Can you work these out from the model? Positions are in its coordinate system, mm. Give positions to 0.01 mm unless a question says otherwise; leave off trailing zeros. Write each loop counter-clockwise with the first axis right and the second up, starting at its lowest first coordinate (ties: lowest second). Pieces come first, ordered by that corner, then holes. Notation, with made-up numbers: (50.5, 4) -> (78.5, 4) arc R20 cw to (78.5, 17) -> close; hole circle Ø11 at (5, 23). An arc over 180 degrees is marked (long way). Answer as CSV lines item,"result". Start each with the question number.
1. If we section it at B-B on x = 1.5: Write out the boundary of the cut face in (y, z), plus the area to 3 significant figures.
2. I need wall thicknesses on line 1 (X direction, y = 0.2, z = -4.5); line 2 (X direction, y = 0.25, z = -1); line 3 (Z direction, x = 0.25, y = 0.3). Which ranges of each line are inside material? Lowest first, please. Write a range as [from, to].
3. If we section it at A-A on z = 1: Write out the boundary of the cut face in (x, y).
4. If we section it at C-C on y = 0.4: Count the separate pieces of the cut face and the enclosed holes in it, plus the area to 3 significant figures.
5. If we section it at D-D on x = -4.5: Write out the boundary of the cut face in (y, z), plus the area to 3 significant figures.
```python
from build123d import *

# Parameters (mm, degrees)
ESQUISSE1_R        = 0.16
BOSS_EXTRU_1_DEPTH = 0.5


with BuildPart() as part:
    # Esquisse1 → Boss.-Extru.1 (new body)
    with BuildSketch(Plane(origin=(0, 0, 0), x_dir=(1, 0, 0), z_dir=(0, 1, 0))):
        with BuildLine():
            ThreePointArc((5.497543289, -0.164370862), (5.499385788, -0.08219461), (5.5, 0))
            ThreePointArc((5.5, 0), (5.499385788, 0.08219461), (5.497543289, 0.164370862))
            ThreePointArc((5.497543289, 0.164370862), (4.96354437, 0.602683401), (5.377131195, 1.15605368))
            ThreePointArc((5.377131195, 1.15605368), (5.340179996, 1.316236154), (5.298458151, 1.475242768))
            ThreePointArc((5.298458151, 1.475242768), (4.675081213, 1.773024435), (4.94421978, 2.409292585))
            ThreePointArc((4.94421978, 2.409292585), (4.870008141, 2.555977446), (4.791445883, 2.700378926))
            ThreePointArc((4.791445883, 2.700378926), (4.114919329, 2.840323734), (4.223968284, 3.522512163))
            ThreePointArc((4.223968284, 3.522512163), (4.116809115, 3.64717462), (4.005972198, 3.768578877))
            ThreePointArc((4.005972198, 3.768578877), (3.315613291, 3.742553741), (3.258235104, 4.431016137))
            ThreePointArc((3.258235104, 4.431016137), (3.124356107, 4.526411262), (2.987685969, 4.617762722))
            ThreePointArc((2.987685969, 4.617762722), (2.32361586, 4.427280128), (2.103145143, 5.082005559))
            ThreePointArc((2.103145143, 5.082005559), (1.950326879, 5.142589335), (1.795766291, 5.198578982))
            ThreePointArc((1.795766291, 5.198578982), (1.196578321, 4.854709087), (0.825828031, 5.437647291))
            ThreePointArc((0.825828031, 5.437647291), (0.662951741, 5.459898808), (0.499483204, 5.477272727))
            ThreePointArc((0.499483204, 5.477272727), (0, 5), (-0.499483204, 5.477272727))
            ThreePointArc((-0.499483204, 5.477272727), (-0.662951741, 5.459898808), (-0.825828031, 5.437647291))
            ThreePointArc((-0.825828031, 5.437647291), (-0.818639901, 5.389149062), (-0.816236154, 5.340179996))
            ThreePointArc((-0.816236154, 5.340179996), (-1.24469969, 4.845323921), (-1.795766291, 5.198578982))
            ThreePointArc((-1.795766291, 5.198578982), (-1.950326879, 5.142589335), (-2.103145143, 5.082005559))
            ThreePointArc((-2.103145143, 5.082005559), (-2.067911799, 4.978598768), (-2.055977446, 4.870008141))
            ThreePointArc((-2.055977446, 4.870008141), (-2.425314256, 4.387382892), (-2.987685969, 4.617762722))
            ThreePointArc((-2.987685969, 4.617762722), (-3.124356107, 4.526411262), (-3.258235104, 4.431016137))
            ThreePointArc((-3.258235104, 4.431016137), (-3.175756675, 4.283437807), (-3.14717462, 4.116809115))
            ThreePointArc((-3.14717462, 4.116809115), (-3.459290066, 3.653452455), (-4.005972198, 3.768578877))
            ThreePointArc((-4.005972198, 3.768578877), (-4.116809115, 3.64717462), (-4.223968284, 3.522512163))
            ThreePointArc((-4.223968284, 3.522512163), (-4.078515354, 3.346593042), (-4.026411262, 3.124356107))
            ThreePointArc((-4.026411262, 3.124356107), (-4.284045125, 2.687024819), (-4.791445883, 2.700378926))
            ThreePointArc((-4.791445883, 2.700378926), (-4.870008141, 2.555977446), (-4.94421978, 2.409292585))
            ThreePointArc((-4.94421978, 2.409292585), (-4.724746794, 2.224931342), (-4.642589335, 1.950326879))
            ThreePointArc((-4.642589335, 1.950326879), (-4.849275857, 1.545398238), (-5.298458151, 1.475242768))
            ThreePointArc((-5.298458151, 1.475242768), (-5.340179996, 1.316236154), (-5.377131195, 1.15605368))
            ThreePointArc((-5.377131195, 1.15605368), (-5.07820272, 0.985919382), (-4.959898808, 0.662951741))
            ThreePointArc((-4.959898808, 0.662951741), (-5.119915162, 0.296330519), (-5.497543289, 0.164370862))
            ThreePointArc((-5.497543289, 0.164370862), (-5.5, 0), (-5.497543289, -0.164370862))
            ThreePointArc((-5.497543289, -0.164370862), (-5.119915162, -0.296330519), (-4.959898808, -0.662951741))
            ThreePointArc((-4.959898808, -0.662951741), (-5.07820272, -0.985919382), (-5.377131195, -1.15605368))
            ThreePointArc((-5.377131195, -1.15605368), (-5.340179996, -1.316236154), (-5.298458151, -1.475242768))
            ThreePointArc((-5.298458151, -1.475242768), (-4.849275857, -1.545398238), (-4.642589335, -1.950326879))
            ThreePointArc((-4.642589335, -1.950326879), (-4.724746794, -2.224931342), (-4.94421978, -2.409292585))
            ThreePointArc((-4.94421978, -2.409292585), (-4.870008141, -2.555977446), (-4.791445883, -2.700378926))
            ThreePointArc((-4.791445883, -2.700378926), (-4.284045125, -2.687024819), (-4.026411262, -3.124356107))
            ThreePointArc((-4.026411262, -3.124356107), (-4.078515354, -3.346593042), (-4.223968284, -3.522512163))
            ThreePointArc((-4.223968284, -3.522512163), (-4.116809115, -3.64717462), (-4.005972198, -3.768578877))
            ThreePointArc((-4.005972198, -3.768578877), (-3.459290066, -3.653452455), (-3.14717462, -4.116809115))
            ThreePointArc((-3.14717462, -4.116809115), (-3.175756675, -4.283437807), (-3.258235104, -4.431016137))
            ThreePointArc((-3.258235104, -4.431016137), (-3.124356107, -4.526411262), (-2.987685969, -4.617762722))
            ThreePointArc((-2.987685969, -4.617762722), (-2.425314256, -4.387382892), (-2.055977446, -4.870008141))
            ThreePointArc((-2.055977446, -4.870008141), (-2.067911799, -4.978598768), (-2.103145143, -5.082005559))
            ThreePointArc((-2.103145143, -5.082005559), (-1.950326879, -5.142589335), (-1.795766291, -5.198578982))
            ThreePointArc((-1.795766291, -5.198578982), (-1.24469969, -4.845323921), (-0.816236154, -5.340179996))
            ThreePointArc((-0.816236154, -5.340179996), (-0.818639901, -5.389149062), (-0.825828031, -5.437647291))
            ThreePointArc((-0.825828031, -5.437647291), (-0.662951741, -5.459898808), (-0.499483204, -5.477272727))
            ThreePointArc((-0.499483204, -5.477272727), (0, -5), (0.499483204, -5.477272727))
            ThreePointArc((0.499483204, -5.477272727), (0.662951741, -5.459898808), (0.825828031, -5.437647291))
            ThreePointArc((0.825828031, -5.437647291), (1.196578321, -4.854709087), (1.795766291, -5.198578982))
            ThreePointArc((1.795766291, -5.198578982), (1.950326879, -5.142589335), (2.103145143, -5.082005559))
            ThreePointArc((2.103145143, -5.082005559), (2.32361586, -4.427280128), (2.987685969, -4.617762722))
            ThreePointArc((2.987685969, -4.617762722), (3.124356107, -4.526411262), (3.258235104, -4.431016137))
            ThreePointArc((3.258235104, -4.431016137), (3.315613291, -3.742553741), (4.005972198, -3.768578877))
            ThreePointArc((4.005972198, -3.768578877), (4.116809115, -3.64717462), (4.223968284, -3.522512163))
            ThreePointArc((4.223968284, -3.522512163), (4.114919329, -2.840323734), (4.791445883, -2.700378926))
            ThreePointArc((4.791445883, -2.700378926), (4.870008141, -2.555977446), (4.94421978, -2.409292585))
            ThreePointArc((4.94421978, -2.409292585), (4.675081213, -1.773024435), (5.298458151, -1.475242768))
            ThreePointArc((5.298458151, -1.475242768), (5.340179996, -1.316236154), (5.377131195, -1.15605368))
            ThreePointArc((5.377131195, -1.15605368), (4.96354437, -0.602683401), (5.497543289, -0.164370862))
        make_face()
        with Locations((0, -4)):
            Circle(ESQUISSE1_R, mode=Mode.SUBTRACT)
        with Locations((-4, 0)):
            Circle(ESQUISSE1_R, mode=Mode.SUBTRACT)
        with BuildLine():
            ThreePointArc((3.8, 0), (-2.687005769, -2.687005769), (0, 3.8))
            ThreePointArc((0, 3.8), (2.687005769, 2.687005769), (3.8, 0))
        make_face(mode=Mode.SUBTRACT)
        with BuildLine():
            ThreePointArc((0.16, 4), (0.113137085, 3.886862915), (0, 3.84))
            ThreePointArc((0, 3.84), (-0.113137085, 4.113137085), (0.16, 4))
        make_face(mode=Mode.SUBTRACT)
        with Locations((4, 0)):
            Circle(ESQUISSE1_R, mode=Mode.SUBTRACT)
    extrude(amount=BOSS_EXTRU_1_DEPTH)


solid = part.part
```
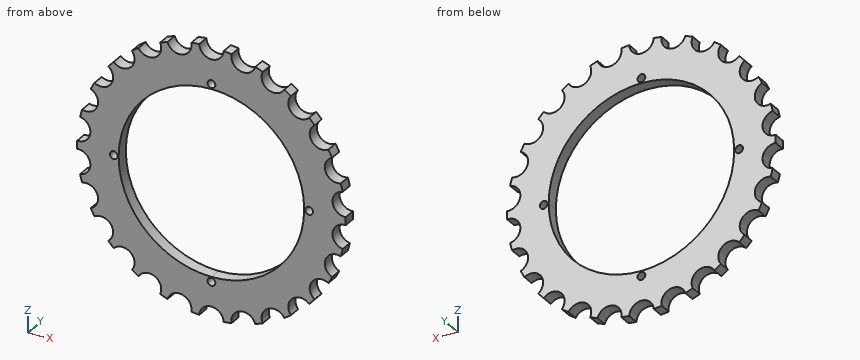
Computed values:
1,outline,"(0, -4.88) -> (0.5, -4.88) -> (0.5, -3.49) -> (0, -3.49) -> close; (0, 3.49) -> (0.5, 3.49) -> (0.5, 4.88) -> (0, 4.88) -> close"
1,area,"1.38 mm2"
2,line 1,"x = [-3.16, -2.89], [-2.22, 2.22], [2.89, 3.16]"
2,line 2,"x = [-5.09, -3.67], [3.67, 5.09]"
2,line 3,"z = [-5.07, -3.79], [3.79, 5.07]"
3,outline,"(-5.09, 0) -> (-3.67, 0) -> (-3.67, 0.5) -> (-5.09, 0.5) -> close; (3.67, 0) -> (5.09, 0) -> (5.09, 0.5) -> (3.67, 0.5) -> close"
4,separate pieces,"1"
4,enclosed holes,"5"
4,area,"39.3 mm2"
5,outline,"(0, -2.63) -> (0.5, -2.63) -> (0.5, 2.63) -> (0, 2.63) -> close"
5,area,"2.63 mm2"
